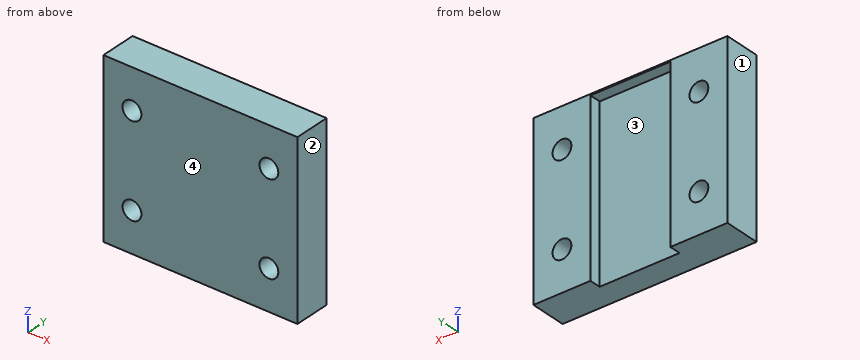
```python
from build123d import *

# Parameters (mm, degrees)
SKETCH1_W           = 34
SKETCH1_H           = 6.35
BOSS_EXTRUDE2_DEPTH = 15
SKETCH3_R           = 1.65
CUT_EXTRUDE1_DEPTH  = 6.35
SKETCH4_W           = 14
SKETCH4_H           = 29.754966952
CUT_EXTRUDE2_DEPTH  = 2


with BuildPart() as part:
    # Sketch1 → Boss-Extrude2 (new body, symmetric)
    with BuildSketch(Plane.XY):
        with Locations((0, 3.175)):
            Rectangle(SKETCH1_W, SKETCH1_H)
    extrude(amount=BOSS_EXTRUDE2_DEPTH, both=True)

    # Sketch3 → Cut-Extrude1 (cut)
    with BuildSketch(Plane.XZ):
        with Locations((-12, 8)):
            Circle(SKETCH3_R)
        with Locations((12, 8)):
            Circle(SKETCH3_R)
        with Locations((-12, -8)):
            Circle(SKETCH3_R)
        with Locations((12, -8)):
            Circle(SKETCH3_R)
    extrude(amount=-CUT_EXTRUDE1_DEPTH, mode=Mode.SUBTRACT)

    # Sketch4 → Cut-Extrude2 (cut)
    with BuildSketch(Plane(origin=(0, 6.35, 0), x_dir=(1, 0, 0), z_dir=(0, 1, 0))):
        with Locations((0, 0.122516524)):
            Rectangle(SKETCH4_W, SKETCH4_H)
    extrude(amount=-CUT_EXTRUDE2_DEPTH, mode=Mode.SUBTRACT)


solid = part.part
```
The model under review builds one solid part; all positions refer to its coordinate system, in mm. Face numbers are marked on the shaded views. Coordinates: 2 decimals unless noted, no trailing zeros. Order: outer loops, then holes, each group sorted by start corner. A loop starts at its lowest first (then second) coordinate and runs counter-clockwise, first axis right, second up. Notation, with made-up numbers: (40.25, 17) -> (60.25, 17) arc R32 ccw to (60.25, 44) -> close; hole circle Ø11 at (0.5, 39.25). An arc over 180 degrees is marked (long way). Answer in a Markdown table with one row per item. Add a question column.
Item 1: Clearance check with flat-ended pins moving along their axes: pin 1 (3 mm diameter, centred on x = 12, z = 8, fed in from +Y); pin 2 (1 mm diameter, centred on x = -2.5, y = 5, fed in from -Z). State where each tip first meets the part, or that it passes through.
Item 2: To check wall thickness, follow probe 1 along Z at (x, y) = (-12, 2); probe 2 along X at (y, z) = (5.5, -1); probe 3 along X at (y, z) = (3.25, 7.5). State the ranges of each line that lie inside material, in increasing order.
Item 3: We need section A-A on x = 12. Write out the cut boundary in (y, z), plus the area to 3 significant figures.
Item 4: We need section B-B on y = 3. Write out the cut boundary in (x, z), plus the area to 3 significant figures.
Item 5: We need section D-D on z = 5.25. Write out the cut boundary in (x, y).
Item 6: We need section C-C on z = -8. Write out the cut boundary in (x, y).
Item 7: Mouldability with a two-part tool opening along X and no side actions: class the marked faces 1, 2, 3 and 4 as +X half, -X half, draft (parallel to the pull), parting line (faces both ways), or undercut.
Final values:
| question | item | result |
|---|---|---|
| 1 | pin 1 | passes through |
| 1 | pin 2 | stops at z = 14.75 |
| 2 | probe 1 | z = -15 to -9.65, -6.35 to 6.35, 9.65 to 15 |
| 2 | probe 2 | x = -17 to -7, 7 to 17 |
| 2 | probe 3 | x = -17 to -13.57, -10.43 to 10.43, 13.57 to 17 |
| 3 | outline | (0, -15) -> (6.35, -15) -> (6.35, -9.65) -> (0, -9.65) -> close; (0, -6.35) -> (6.35, -6.35) -> (6.35, 6.35) -> (0, 6.35) -> close; (0, 9.65) -> (6.35, 9.65) -> (6.35, 15) -> (0, 15) -> close |
| 3 | area | 149 mm2 |
| 4 | outline | (-17, -15) -> (17, -15) -> (17, 15) -> (-17, 15) -> close; hole circle Ø3.3 at (-12, -8); hole circle Ø3.3 at (-12, 8); hole circle Ø3.3 at (12, -8); hole circle Ø3.3 at (12, 8) |
| 4 | area | 986 mm2 |
| 5 | outline | (-17, 0) -> (17, 0) -> (17, 6.35) -> (7, 6.35) -> (7, 4.35) -> (-7, 4.35) -> (-7, 6.35) -> (-17, 6.35) -> close |
| 6 | outline | (-17, 0) -> (-13.65, 0) -> (-13.65, 6.35) -> (-17, 6.35) -> close; (-10.35, 0) -> (10.35, 0) -> (10.35, 6.35) -> (7, 6.35) -> (7, 4.35) -> (-7, 4.35) -> (-7, 6.35) -> (-10.35, 6.35) -> close; (13.65, 0) -> (17, 0) -> (17, 6.35) -> (13.65, 6.35) -> close |
| 7 | face 1 | -X half |
| 7 | face 2 | +X half |
| 7 | face 3 | undercut |
| 7 | face 4 | draft |
